Part model, mm, in its own coordinate system. A direction names the side the tool comes from. Round coordinates to 2 decimals unless told otherwise and drop trailing zeros. Loops run counter-clockwise (first coordinate to the right, second up) from the corner with the lowest first, then second, coordinate; pieces in that order, holes last.
(1) Cut at C-C on x = -34.5. List the corners of the cut face in (y, z), then the cut area to 3 significant figures.
(2) Flat gauge pins, fed straight in: pin 1 (10 mm diameter, centred on y = 16.5, z = -13.5, fed in from -X); pin 2 (12 mm diameter, centred on x = -3.5, z = -30.5, fed in from +Y); pin 3 (8.5 mm diameter, centred on y = 13.5, z = -9.5, fed in from +X). Where does each tip first touch, or does it go through?
(3) Probe probe 1 along X at (y, z) = (0.5, -24.5); probe 2 along Z at (x, y) = (-13.5, 19); probe 3 along X at (y, z) = (8, 31). List the from-to ranges inside material, lowest first.
(4) Tool access for faces 4 (the face through (-4, 0, 38)), 5 (the face through (-54, 19.15, -38)), 6 (the face through (-9, 1, -30.5)), 7 (the face through (-48.5, 15, 1)), 8 (the face through (54, 8.85, -38)): list every direction of +Z, -Z, +X, -X, +Y, -Y with a clear straight run to the whole face (end or side of a thin tool).
(5) Mould opens along Z. For faces 1 (the face through (-58, 14, -38)), 2 (the face through (-56, 13, -35)), 3 (the face through (-35.4, 0.5, 23.3)) say: +Z half, -Z half, draft (parallel to the pull), parting line (faces both ways), or undercut.
(6) Cut at B-B on x = 34.5. List the corners of the cut face in (y, z), then the cut area to 3 significant figures.
(7) Cut at D-D on z = -0.5. List the corners of the cut face in (x, y).
(8) Cut at A-A on z = -24.5. List the corners of the cut face in (x, y), then the cut area to 3 significant figures.
from build123d import *

# Parameters (mm, degrees)
SKETCH1_W           = 100
SKETCH1_H           = 80
BOSS_EXTRUDE1_DEPTH = 3
SKETCH2_W           = 100
SKETCH2_H           = 80
SKETCH2_W_2         = 97
SKETCH2_H_2         = 77.6
BOSS_EXTRUDE2_DEPTH = 25
SKETCH3_R           = 1.5
CUT_EXTRUDE1_DEPTH  = 40
SKETCH4_W           = 95
SKETCH4_H           = 75
BOSS_EXTRUDE3_DEPTH = 5
SKETCH3_2_R         = 1.5
CUT_EXTRUDE2_DEPTH  = 12
SKETCH6_W           = 8
SKETCH6_H           = 10.3
SKETCH6_R           = 2
BOSS_EXTRUDE4_DEPTH = 5
FILLET1_R           = 1
FILLET2_R           = 1
FILLET3_R           = 1
FILLET4_R           = 1
FILLET5_R           = 1
FILLET6_R           = 1
FILLET7_R           = 1
FILLET8_R           = 1
FILLET9_R           = 1
FILLET10_R          = 1


with BuildPart() as part:
    # Sketch1 → Boss-Extrude1 (new body)
    with BuildSketch(Plane(origin=(0, 0, 0), x_dir=(1, 0, 0), z_dir=(0, 1, 0))):
        Rectangle(SKETCH1_W, SKETCH1_H)
    extrude(amount=BOSS_EXTRUDE1_DEPTH)

    # Sketch2 → Boss-Extrude2 (add)
    with BuildSketch(Plane(origin=(0, 3, 0), x_dir=(1, 0, 0), z_dir=(0, 1, 0))):
        Rectangle(SKETCH2_W, SKETCH2_H)
        Rectangle(SKETCH2_W_2, SKETCH2_H_2, mode=Mode.SUBTRACT)
    extrude(amount=BOSS_EXTRUDE2_DEPTH)

    # Sketch3 → Cut-Extrude1 (cut)
    with BuildSketch(Plane(origin=(0, 3, 0), x_dir=(1, 0, 0), z_dir=(0, 1, 0))):
        with Locations(Location((-34.5, 24.5, 0), (0, 0, 270))):
            Circle(SKETCH3_R)
        with Locations(Location((34.5, 24.5, 0), (0, 0, 270))):
            Circle(SKETCH3_R)
        with Locations(Location((-34.5, -24.5, 0), (0, 0, 270))):
            Circle(SKETCH3_R)
        with Locations(Location((34.5, -24.5, 0), (0, 0, 270))):
            Circle(SKETCH3_R)
        with BuildLine():
            Line((-39.5, 38.5), (20.5, 38.5))
            ThreePointArc((20.5, 38.5), (24.5, 34.5), (20.5, 30.5))
            Line((20.5, 30.5), (-39.5, 30.5))
            ThreePointArc((-39.5, 30.5), (-43.5, 34.5), (-39.5, 38.5))
        make_face()
    extrude(amount=-CUT_EXTRUDE1_DEPTH, mode=Mode.SUBTRACT)

    # Sketch4 → Boss-Extrude3 (add)
    with BuildSketch(Plane(origin=(0, 3, 0), x_dir=(1, 0, 0), z_dir=(0, 1, 0))):
        Rectangle(SKETCH4_W, SKETCH4_H)
    extrude(amount=-BOSS_EXTRUDE3_DEPTH)

    # Sketch3_2 → Cut-Extrude2 (cut)
    with BuildSketch(Plane(origin=(0, 3, 0), x_dir=(1, 0, 0), z_dir=(0, 1, 0))):
        with Locations(Location((-34.5, 24.5, 0), (0, 0, 270))):
            Circle(SKETCH3_2_R)
        with Locations(Location((34.5, 24.5, 0), (0, 0, 270))):
            Circle(SKETCH3_2_R)
        with Locations(Location((-34.5, -24.5, 0), (0, 0, 270))):
            Circle(SKETCH3_2_R)
        with Locations(Location((34.5, -24.5, 0), (0, 0, 270))):
            Circle(SKETCH3_2_R)
        with BuildLine():
            Line((-39.5, 38.5), (20.5, 38.5))
            ThreePointArc((20.5, 38.5), (24.5, 34.5), (20.5, 30.5))
            Line((20.5, 30.5), (-39.5, 30.5))
            ThreePointArc((-39.5, 30.5), (-43.5, 34.5), (-39.5, 38.5))
        make_face()
    extrude(amount=-CUT_EXTRUDE2_DEPTH, mode=Mode.SUBTRACT)

    # Sketch6 → Boss-Extrude4 (add)
    # profile 1 of 2: a face of its own
    with BuildSketch(Plane(origin=(0, 0, -40), x_dir=(-1, 0, 0), z_dir=(0, 0, -1))):
        with Locations((-54, 14)):
            Rectangle(SKETCH6_W, SKETCH6_H)
        with Locations((-54, 14)):
            Circle(SKETCH6_R, mode=Mode.SUBTRACT)
    # profile 2 of 2: a face of its own
    with BuildSketch(Plane(origin=(0, 0, -40), x_dir=(-1, 0, 0), z_dir=(0, 0, -1))):
        with Locations((54, 14)):
            Rectangle(SKETCH6_W, SKETCH6_H)
        with Locations((54, 14)):
            Circle(SKETCH6_R, mode=Mode.SUBTRACT)
    extrude(amount=-BOSS_EXTRUDE4_DEPTH)

    # Fillet1
    fillet1_edges = [part.edges().sort_by_distance(p)[0] for p in [
        (50, 8.85, -37.5),
    ]]
    fillet(fillet1_edges, radius=FILLET1_R)

    # Fillet2
    fillet2_edges = [part.edges().sort_by_distance(p)[0] for p in [
        (58, 8.85, -37.5),
    ]]
    fillet(fillet2_edges, radius=FILLET2_R)

    # Fillet3
    fillet3_edges = [part.edges().sort_by_distance(p)[0] for p in [
        (58, 19.15, -37.5),
    ]]
    fillet(fillet3_edges, radius=FILLET3_R)

    # Fillet4
    fillet4_edges = [part.edges().sort_by_distance(p)[0] for p in [
        (50, 19.15, -37.5),
    ]]
    fillet(fillet4_edges, radius=FILLET4_R)

    # Fillet5
    fillet5_edges = [part.edges().sort_by_distance(p)[0] for p in [
        (50, 14, -35),
    ]]
    fillet(fillet5_edges, radius=FILLET5_R)

    # Fillet6
    fillet6_edges = [part.edges().sort_by_distance(p)[0] for p in [
        (-58, 8.85, -37.5),
    ]]
    fillet(fillet6_edges, radius=FILLET6_R)

    # Fillet7
    fillet7_edges = [part.edges().sort_by_distance(p)[0] for p in [
        (-58, 19.15, -37.5),
    ]]
    fillet(fillet7_edges, radius=FILLET7_R)

    # Fillet8
    fillet8_edges = [part.edges().sort_by_distance(p)[0] for p in [
        (-50, 19.15, -37.5),
    ]]
    fillet(fillet8_edges, radius=FILLET8_R)

    # Fillet9
    fillet9_edges = [part.edges().sort_by_distance(p)[0] for p in [
        (-50, 8.85, -37.5),
    ]]
    fillet(fillet9_edges, radius=FILLET9_R)

    # Fillet10
    fillet10_edges = [part.edges().sort_by_distance(p)[0] for p in [
        (-50, 14, -35),
    ]]
    fillet(fillet10_edges, radius=FILLET10_R)


solid = part.part
Final values:
1. outline: (-2, -30.5) - (3, -30.5) - (3, -26) - (-2, -26) - close; (-2, -23) - (3, -23) - (3, 23) - (-2, 23) - close; (-2, 26) - (3, 26) - (3, 38.8) - (28, 38.8) - (28, 40) - (0, 40) - (0, 37.5) - (-2, 37.5) - close; (0, -40) - (28, -40) - (28, -38.8) - (3, -38.8) - (3, -38.5) - (0, -38.5) - close
1. area: 382 mm2
2. pin 1: stops at x = -50
2. pin 2: stops at y = 3
2. pin 3: stops at x = 50
3. probe 1: x = -50 to -36, -33 to 33, 36 to 50
3. probe 2: z = -40 to -38.8, 38.8 to 40
3. probe 3: x = -50 to -48.5, 48.5 to 50
4. face 4: -Y
4. face 5: +Z, -Z, -X, +Y
4. face 6: +Y, -Y
4. face 7: +Y
4. face 8: +Z, -Z, +X, -Y
5. face 1: draft
5. face 2: +Z half
5. face 3: undercut
6. outline: (-2, -37.5) - (0, -37.5) - (0, -40) - (28, -40) - (28, -38.8) - (3, -38.8) - (3, -26) - (-2, -26) - close; (-2, -23) - (3, -23) - (3, 23) - (-2, 23) - close; (-2, 26) - (3, 26) - (3, 38.8) - (28, 38.8) - (28, 40) - (0, 40) - (0, 37.5) - (-2, 37.5) - close
6. area: 420 mm2
7. outline: (-50, 0) - (-47.5, 0) - (-47.5, -2) - (47.5, -2) - (47.5, 0) - (50, 0) - (50, 28) - (48.5, 28) - (48.5, 3) - (-48.5, 3) - (-48.5, 28) - (-50, 28) - close
8. outline: (-50, 0) - (-47.5, 0) - (-47.5, -2) - (-36, -2) - (-36, 3) - (-48.5, 3) - (-48.5, 28) - (-50, 28) - close; (-33, -2) - (33, -2) - (33, 3) - (-33, 3) - close; (36, -2) - (47.5, -2) - (47.5, 0) - (50, 0) - (50, 28) - (48.5, 28) - (48.5, 3) - (36, 3) - close
8. area: 535 mm2
